Can you work these out from the model? Positions are in its coordinate system, mm. Face numbers are marked on the shaded views. A direction names the side the tool comes from. Give positions to 0.01 mm unless a question says otherwise; leave off trailing zeros. Loops run counter-clockwise (first coordinate to the right, second up) from the corner with the lowest first, then second, coordinate; pieces in that order, holes last. Notation, with made-up numbers: (81.5, 30.5) - (123.5, 30.5) arc R31 cw to (123.5, 65.5) - close; hole circle Ø10 at (1, 41.5). An arc over 180 degrees is marked (long way). Use a Markdown table: item, result. Add a question column.
```python
from build123d import *

# Parameters (mm, degrees)
ESQUISSE1_R             = 22
BOSS_EXTRU_1_DEPTH      = 50
BOSS_EXTRU_3_DEPTH      = 20.2
BOSS_EXTRU_3_DEPTH_BACK = 20.2
ENL_V_MAT_EXTRU_1_REACH = 100.801
ESQUISSE6_R             = 15
ENL_V_MAT_EXTRU_2_DEPTH = 10.3
ENL_V_MAT_EXTRU_3_REACH = 100.406
ESQUISSE7_R             = 12.75
CONG_1_R                = 1
ESQUISSE8_R             = 18
ENL_V_MAT_EXTRU_4_DEPTH = 2
ENL_V_START             = -15.6
ENL_V_MAT_EXTRU_5_DEPTH = 15.6
CONG_5_R                = 1


with BuildPart() as part:
    # Esquisse1 → Boss.-Extru.1 (new body)
    with BuildSketch(Plane.XY):
        Circle(ESQUISSE1_R)
    extrude(amount=BOSS_EXTRU_1_DEPTH)

    # Esquisse4 → Boss.-Extru.3 (add, two sides: drawn at the far end of the back side and taken through both)
    with BuildSketch(Plane.XZ.offset(-BOSS_EXTRU_3_DEPTH_BACK)):
        Polygon((-35.991735162, 60.008264838), (-50.275292142, 74.291821818), (-61.306157929, 63.260956031), (-22, 23.954798102), (0, 23.954798102), (0, 46.016529675), (-22, 46.016529675), align=None)
    extrude(amount=BOSS_EXTRU_3_DEPTH + BOSS_EXTRU_3_DEPTH_BACK)

    # Esquisse5 → Enlèv. mat.-Extru.1 (cut, up to next)
    with BuildSketch(Plane(origin=(0, 0, 0), x_dir=(-1, 0, 0), z_dir=(0, 0, -1)), mode=Mode.PRIVATE) as enl_v_mat_extru_1_sk1:
        with BuildLine():
            Line((-12.8, -6), (-12.8, 6))
            Line((-12.8, 6), (-8, 6))
            ThreePointArc((-8, 6), (10, 0), (-8, -6))
            Line((-8, -6), (-12.8, -6))
        make_face()
    enl_v_mat_extru_1_tool1 = extrude(enl_v_mat_extru_1_sk1.sketch, amount=-ENL_V_MAT_EXTRU_1_REACH, mode=Mode.PRIVATE) & part.part
    add(enl_v_mat_extru_1_tool1.solids().sort_by_distance((1.280327, 0, 0))[0], mode=Mode.SUBTRACT)

    # Esquisse6 → Enlèv. mat.-Extru.2 (cut)
    with BuildSketch(Plane(origin=(12.008264838, 0, 12.008264838), x_dir=(0.7071067811865508, 0, -0.7071067811865444), z_dir=(0.7071067811865444, 0, 0.7071067811865508))):
        with Locations((-67.882250994, 0)):
            Circle(ESQUISSE6_R)
    extrude(amount=-ENL_V_MAT_EXTRU_2_DEPTH, mode=Mode.SUBTRACT)

    # Esquisse7 → Enlèv. mat.-Extru.3 (cut, up to next)
    with BuildSketch(Plane(origin=(4.725064991, 0, 4.725064991), x_dir=(0.7071067811865507, 0, -0.7071067811865445), z_dir=(0.7071067811865445, 0, 0.7071067811865507)), mode=Mode.PRIVATE) as enl_v_mat_extru_3_sk1:
        with Locations((-67.882250994, 0)):
            Circle(ESQUISSE7_R)
    enl_v_mat_extru_3_tool1 = extrude(enl_v_mat_extru_3_sk1.sketch, amount=-ENL_V_MAT_EXTRU_3_REACH, mode=Mode.PRIVATE) & part.part
    add(enl_v_mat_extru_3_tool1.solids().sort_by_distance((-43.274935, 0, 52.725065))[0], mode=Mode.SUBTRACT)

    # Congé1
    cong_1_edges = [part.edges().sort_by_distance(p)[0] for p in [
        (-56.038212409, 0, 57.993010511),
    ]]
    fillet(cong_1_edges, radius=CONG_1_R)

    # Esquisse8 → Enlèv. mat.-Extru.4 (cut)
    with BuildSketch(Plane(origin=(0, 0, 0), x_dir=(-1, 0, 0), z_dir=(0, 0, -1))):
        Circle(ESQUISSE8_R)
    extrude(amount=-ENL_V_MAT_EXTRU_4_DEPTH, mode=Mode.SUBTRACT)

    # Esquisse10 → Enlèv. mat.-Extru.5 (cut)
    with BuildSketch(Plane(origin=(12.008264838, 0, 12.008264838), x_dir=(0.7071067811865509, 0, -0.7071067811865442), z_dir=(0.7071067811865442, 0, 0.7071067811865509)).offset(ENL_V_START)):
        with BuildLine():
            Line((-67.882250994, 20.2), (-92.882250994, 20.2))
            Line((-92.882250994, 20.2), (-92.882250994, -20.2))
            Line((-92.882250994, -20.2), (-67.882250994, -20.2))
            ThreePointArc((-67.882250994, -20.2), (-88.082250994, 0), (-67.882250994, 20.2))
        make_face()
    extrude(amount=ENL_V_MAT_EXTRU_5_DEPTH, mode=Mode.SUBTRACT)

    # Congé5
    cong_5_edges = [part.edges().sort_by_distance(p)[0] for p in [
        (-15.357751714, 20.2, 23.954798102),
        (-15.357751714, -20.2, 23.954798102),
        (-15.357751714, -20.2, 46.016529675),
        (-28.995867581, -20.2, 53.012397256),
        (-28.995867581, 20.2, 53.012397256),
        (-22, 0, 0),
        (-22, 0, 50),
        (-34.511300474, -20.2, 36.466098577),
        (-50.275292142, 0, 74.291821818),
        (-61.306157929, 0, 63.260956031),
        (-34.511300474, 20.2, 36.466098577),
        (-15.357751714, 20.2, 46.016529675),
    ]]
    fillet(cong_5_edges, radius=CONG_5_R)


solid = part.part
```
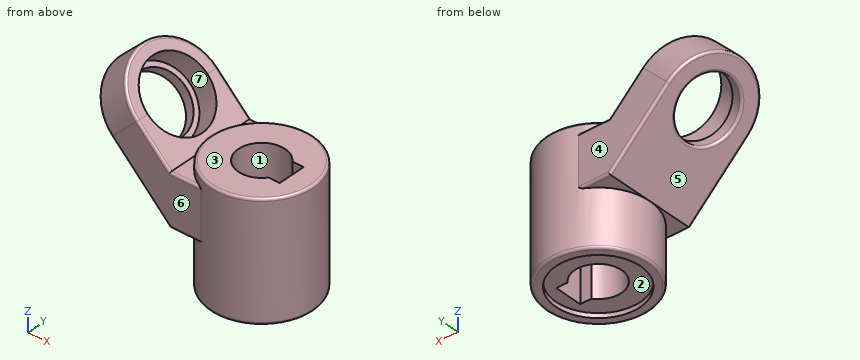
1. Suppose I cut it at A-A (x = 0). List the corners of the cut face in (y, z) for me.
2. On a 3-axis mill with a long thin cutter (end or side, diameter ignored), from which of +Z, -Z, +X, -X, +Y, -Y can I reach the whole of each face in a straight line? I mean the marked faces 1, 2, 3 and 4. Say none if no direction works.
3. Please list where these lines run through material, in increasing order: line 1 along Y through (x, z) = (0, 17.5); line 2 along Y through (x, z) = (0, 1); line 3 along Z through (x, y) = (13.5, 9). Write a range as [from, to].
4. Will these pins go through, and if not, where does the flat tip stop? P1, Ø2, axis at x = -44, y = -14, coming from the -Z side; P2, Ø2, axis at y = 5, z = 31, coming from the -X side; P3, Ø18, axis at x = -2, y = -7.5, coming from the -Z side; P4, Ø12, axis at x = 0, y = 0, coming from the +Z side.
5. Suppose I cut it at B-B (y = 5). State how many separate pieces and enclosed holes the cut face has, and give its area (3 significant figures).
6. If we mould it in two halves opening along X, with no side actions, what happens to the marked faces 5, 6 and 7? For each: released by +X, released by -X, zero draft, split by the parting line, or undercut.
Results below:
| question | item | result |
|---|---|---|
| 1 | outline | (-22, 1) arc R1 ccw to (-21, 0) - (-18, 0) - (-18, 2) - (-10, 2) - (-10, 50) - (-21, 50) arc R1 ccw to (-22, 49) - close; (10, 2) - (18, 2) - (18, 0) - (21, 0) arc R1 ccw to (22, 1) - (22, 49) arc R1 ccw to (21, 50) - (10, 50) - close |
| 2 | face 1 | +Z, -Z |
| 2 | face 2 | -Z |
| 2 | face 3 | +Z, +X, +Y, -Y |
| 2 | face 4 | +Z, -Z, -X, +Y |
| 3 | line 1 | [-22, -10], [10, 22] |
| 3 | line 2 | [-22, -18], [18, 22] |
| 3 | line 3 | [2, 50] |
| 4 | P1 | z = 44.95 |
| 4 | P2 | x = -30.05 |
| 4 | P3 | z = 2 |
| 4 | P4 | through |
| 5 | separate pieces | 3 |
| 5 | enclosed holes | 0 |
| 5 | area | 1,370 mm² |
| 6 | face 5 | released by -X |
| 6 | face 6 | zero draft |
| 6 | face 7 | undercut |
